Autodesk Inventor part; units mm, degrees
ref_plane "Work Plane1" through (-15, -58.5, -186) normal (0, 0, -1) x (0, 1, 0)
ref_plane "YZ Plane" through (0, 0, 0) normal (1, 0, 0) x (0, 1, 0)
ref_plane "XZ Plane" through (0, 0, 0) normal (0, 1, 0) x (-1, 0, 0)
sketch "Sketch1" plane through (0, 0, 0) normal (0, 0, 1) x (1, 0, 0)
  line L0 (7.0071, 53.5071) -> (-15, 31.5) construction
  line L1 (7, 58.5) -> (7, 55.5) construction
  line L2 (7, 57.7426) -> (-15, 35.7426)
  line L3 (-15, 35.7426) -> (-12.8787, 33.6213)
  line L4 (-12.8787, 33.6213) -> (7, 53.5)
  line L5 (7, 53.5) -> (7, 57.7426)
  line L6 (15, 58.5) -> (15, 66.5) construction
  point P0 (0, 0)
  point P1 (15, 62.5)
  dimension "d0" = 30
  dimension "d1" = 3
ref_plane "Work Plane1" through (-15, -58.5, -186) normal (0, 0, -1) x (0, 1, 0)
extrude "Extrusion1" add sketch "Sketch1" against normal up to surface (186 mm away)
ref_plane "Work Plane2" through (1.4452, 43.5974, -13.2717) normal (-0.03, 0.9995, 0) x (0.9995, 0.03, 0)
sketch "Sketch2" plane through (1.4452, 43.5974, -13.2717) normal (-0.03, 0.9995, 0) x (0.9995, 0.03, 0)
  line L0 (-4, 22) -> (-4, 0) construction
  line L1 (4, 22) -> (-4, 22) construction
  line L2 (-4, 0) -> (4, 0) construction
  line L3 (-6, 0) -> (-6, 22)
  line L4 (-4, 24) -> (5.9769, 24)
  line L5 (5.9769, 24) -> (5.9769, -2)
  line L6 (5.9769, -2) -> (-4, -2)
  line L7 (5.9769, 172.7283) -> (-16.6735, 172.7283) construction
  line L8 (-16.6735, -13.2717) -> (-16.6735, 172.7283) construction
  line L9 (5.9769, -13.2717) -> (-16.6735, -13.2717) construction
  line L10 (5.9769, -13.2717) -> (5.9769, 172.7283) construction
  arc A0 (-6, 0) -> (-4, -2) centre (-4, 0) ccw
  arc A1 (-4, 24) -> (-6, 22) centre (-4, 22) ccw
  line L11 (5.9769, 79.7283) -> (-16.6735, 79.7283)
  line L12 (-6, 159.4566) -> (-6, 137.4566)
  line L13 (-4, 135.4566) -> (5.9769, 135.4566)
  line L14 (5.9769, 135.4566) -> (5.9769, 161.4566)
  line L15 (5.9769, 161.4566) -> (-4, 161.4566)
  arc A2 (-4, 161.4566) -> (-6, 159.4566) centre (-4, 159.4566) ccw
  arc A3 (-6, 137.4566) -> (-4, 135.4566) centre (-4, 137.4566) ccw
  point P0 (-2.7531, -13.2717)
  dimension "d4" = 2
  dimension "d5" = 2
  dimension "d6" = 2
  dimension "d7" = 2
  dimension "d8" = 2
extrude "Extrusion2" cut sketch "Sketch2" along normal through all
sketch "Sketch3" plane through (-15, 35.7426, -186) normal (-0.7071, 0.7071, 0) x (-0.7071, -0.7071, 0)
  circle A0 centre (-9.0711, 178) radius 2.25
  circle A1 centre (-18.1127, 178) radius 2.25
  circle A2 centre (-9.0711, 8) radius 2.25
  circle A3 centre (-18.1127, 8) radius 2.25
  point P0 (14.6673, 186)
hole "Hole1" at (-8.5858, 42.1569, -8) at (-2.1924, 48.5503, -8) at (-8.5858, 42.1569, -178) at (-2.1924, 48.5503, -178) direction (0.7071, -0.7071, 0) diameter 3.4 end through all countersink diameter 6.3 countersink angle 90
equation "\"d5\" = d4"
equation "\"d6\" = d4"
properties part number "Przod"
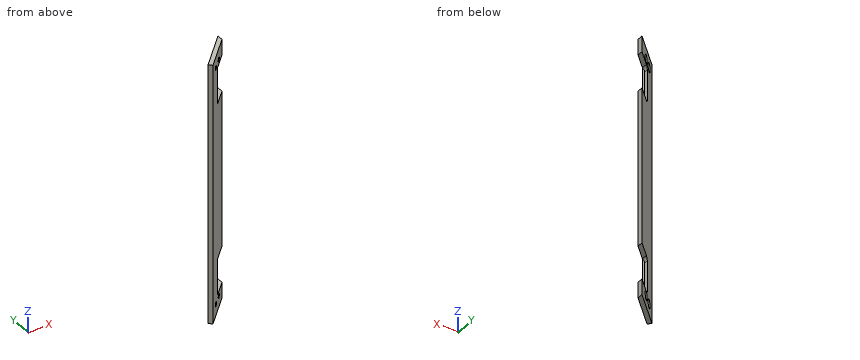
Could you check a few things on this model? Use its own coordinates, in mm. Coordinates: 2 decimals unless noted, no trailing zeros. Loops run counter-clockwise (first coordinate to the right, second up) from the corner with the lowest first, then second, coordinate; pieces in that order, holes last. Notation, with made-up numbers: M 76,9 L 85,9 A18 cw 85,39 Z; hole C -28.5,30 d1. An arc over 180 degrees is marked long. Put each result on its own line as item: value. Start each with the question number.
(1) Suppose I cut it at C-C on z = -135. Please give me the cut outline in (x, y), then the cut area to 3 significant figures.
(2) I need wall thicknesses on line 1 (Z direction, x = 5, y = 53); line 2 (X direction, y = 45.75, z = -47.5); line 3 (X direction, y = 45.25, z = -144). Which ranges of each line are inside material? Lowest first, please. Write a range as from..to.
(3) Suppose I cut it at A-A on x = 5.25. Please give me the cut outline in (y, z).
(4) Suppose I cut it at B-B on z = -166.5. Please give me the cut outline in (x, y), then the cut area to 3 significant figures.
(5) Will these pins go through, and if not, where does the flat tip stop? P1, Ø1, axis at y = 45.5, z = -24, coming from the +X side; P2, Ø5, axis at y = 54.5, z = -125.5, coming from the -X side; P3, Ø5, axis at y = 46.5, z = -94.5, coming from the -X side.
Solutions:
1. outline: M -15,35.74 L -12.88,33.62 L 7,53.5 L 7,57.74 Z
1. area: 88.8 mm2
2. line 1: z = -186..-174.73, -148.73..-37.27, -11.27..0
2. line 2: x = -4.99..-0.75
2. line 3: x = -5.49..-1.25
3. outline: M 51.75,-186 L 55.99,-186 L 55.99,-174.73 L 51.75,-174.73 Z; M 51.75,-148.73 L 55.99,-148.73 L 55.99,-37.27 L 51.75,-37.27 Z; M 51.75,-11.27 L 55.99,-11.27 L 55.99,0 L 51.75,0 Z
4. outline: M -15,35.74 L -12.88,33.62 L -3.04,43.46 L -4.55,43.42 L -4.63,46.11 Z
4. area: 40.8 mm2
5. P1: stops at x = -4.6
5. P2: stops at x = 1.26
5. P3: stops at x = -6.74
